Source: three-view drawing plus pictorial views. Frame: mm from the lowest corner of the part. Give positions to 0.01 mm unless a question says otherwise; leave off trailing zeros. Write each loop counter-clockwise with the first axis right and the second up, starting at its lowest first coordinate (ties: lowest second). Pieces come first, ordered by that corner, then holes. Notation, with made-up numbers: (80, 27) -> (109, 27) arc R25 cw to (109, 64) -> close; hole circle Ø2 at (-39, 60). An arc over 180 degrees is marked (long way). Answer in a Markdown table with one row per item. Add a question column.
Item 1: Section query A-A on z = 17.5. Output: boundary loops of the cut face in (x, y), plus the area to 3 significant figures.
Item 2: Section query D-D on z = 23.25. Output: boundary loops of the cut face in (x, y).
Item 3: Draft query along Y for the marked faces 1, 2, 3 and 4. Return one class per face: +Y half, -Y half, draft (parallel to the pull), parting line (faces both ways), or undercut.
Item 4: Section query C-C on y = 10.75. Output: boundary loops of the cut face in (x, z), plus the area to 3 significant figures.
Item 5: Section query B-B on x = 10. Output: boundary loops of the cut face in (y, z), plus the area to 3 significant figures.
Item 6: First-contact query: P1, Ø8, axis at y = 10, z = 23, coming from the +X side; P2, Ø2, axis at x = 17, y = 4, coming from the +Z side; P3, Ø4, axis at x = 14, y = 10, coming from the +Z side; P4, Ø1, axis at x = 11, y = 4.5, coming from the +Z side. Flat tips, straight axial feed; report the tip coordinate or a pass-through.
Item 7: Material intervals for probe 1 along Y at (x, z) = (16.75, 26.5); probe 2 along Z at (x, y) = (2.75, 11.75); probe 3 along Z at (x, y) = (11.5, 3.25), sorted ascending. Write a range as from..to.
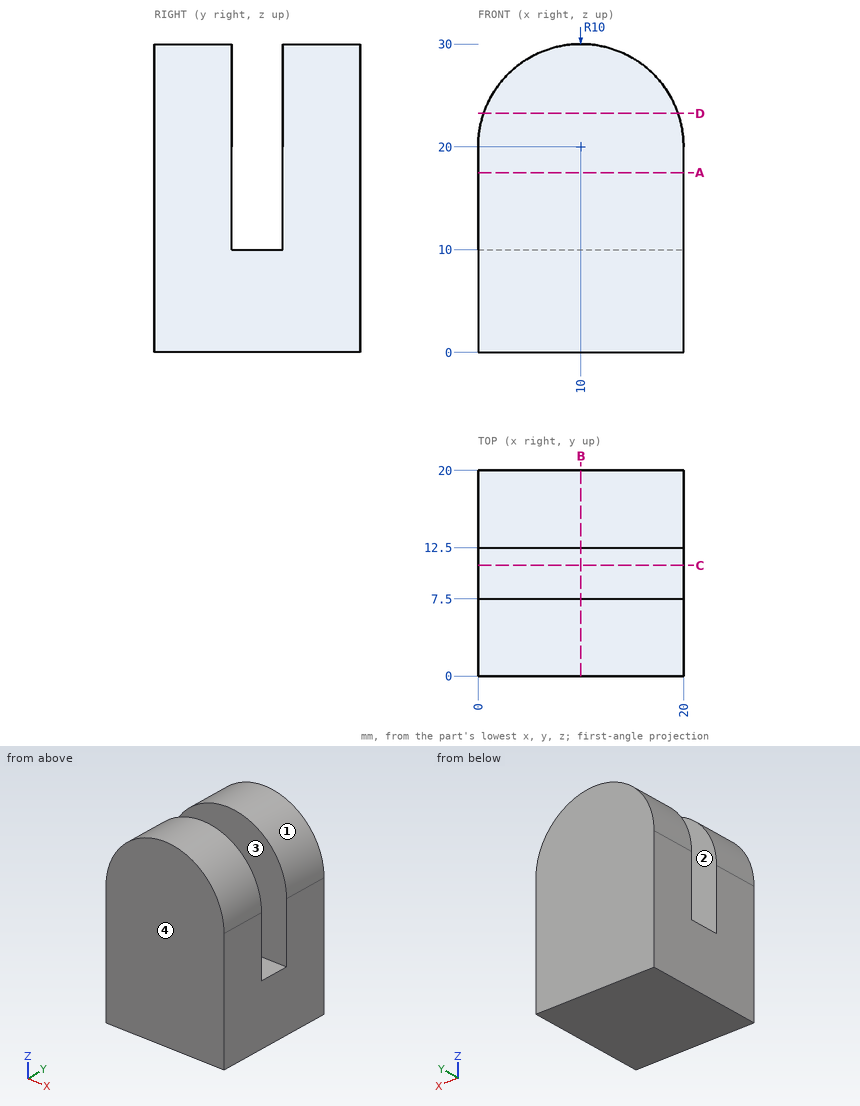
Findings below:
| question | item | result |
|---|---|---|
| 1 | outline | (0, 0) -> (20, 0) -> (20, 7.5) -> (0, 7.5) -> close; (0, 12.5) -> (20, 12.5) -> (20, 20) -> (0, 20) -> close |
| 1 | area | 300 mm^2 |
| 2 | outline | (0.54, 0) -> (19.46, 0) -> (19.46, 7.5) -> (0.54, 7.5) -> close; (0.54, 12.5) -> (19.46, 12.5) -> (19.46, 20) -> (0.54, 20) -> close |
| 3 | face 1 | draft |
| 3 | face 2 | undercut |
| 3 | face 3 | undercut |
| 3 | face 4 | -Y half |
| 4 | outline | (0, 0) -> (20, 0) -> (20, 10) -> (0, 10) -> close |
| 4 | area | 200 mm^2 |
| 5 | outline | (0, 0) -> (20, 0) -> (20, 30) -> (12.5, 30) -> (12.5, 10) -> (7.5, 10) -> (7.5, 30) -> (0, 30) -> close |
| 5 | area | 500 mm^2 |
| 6 | P1 | stops at x = 20 |
| 6 | P2 | stops at z = 28 |
| 6 | P3 | stops at z = 10 |
| 6 | P4 | stops at z = 29.99 |
| 7 | probe 1 | y = 0..7.5, 12.5..20 |
| 7 | probe 2 | z = 0..10 |
| 7 | probe 3 | z = 0..29.89 |
